CAD build for the part. Positions are in the model's coordinates, mm. Face numbers are marked on the shaded views. A direction names the side the tool comes from. Coordinates: 2 decimals unless noted, no trailing zeros. Write each loop counter-clockwise with the first axis right and the second up, starting at its lowest first coordinate (ties: lowest second). Pieces come first, ordered by that corner, then holes.
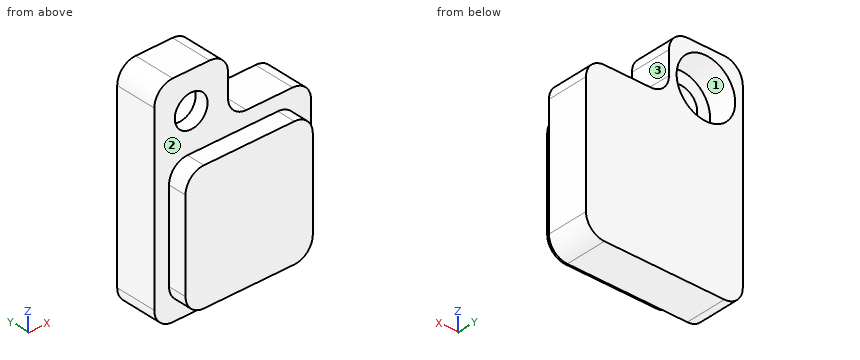
```python
from build123d import *

# Parameters (mm, degrees)
SKETCH1_W                                      = 8.5
SKETCH1_H                                      = 8.5
EXTRUDE1_DEPTH                                 = 2.25
SKETCH7_W                                      = 6.9
SKETCH7_H                                      = 6.9
EXTRUDE5_DEPTH                                 = 1
SKETCH3_W                                      = 4
SKETCH3_H                                      = 2.25
EXTRUDE3_DEPTH                                 = 3.25
CBORE_FOR_0_SOCKET_HEAD_CAP_SCREW1_D           = 1.778
CBORE_FOR_0_SOCKET_HEAD_CAP_SCREW1_CBORE_D     = 3.175
CBORE_FOR_0_SOCKET_HEAD_CAP_SCREW1_CBORE_DEPTH = 1.524
FILLET2_R                                      = 1


with BuildPart() as part:
    # Sketch1 → Extrude1 (new body)
    with BuildSketch(Plane(origin=(0, 0, 0), x_dir=(1, 0, 0), z_dir=(0, 1, 0))):
        Rectangle(SKETCH1_W, SKETCH1_H)
    extrude(amount=EXTRUDE1_DEPTH)

    # Sketch7 → Extrude5 (add)
    with BuildSketch(Plane.XZ):
        Rectangle(SKETCH7_W, SKETCH7_H)
    extrude(amount=EXTRUDE5_DEPTH)

    # Sketch3 → Extrude3 (add)
    with BuildSketch(Plane.XY.offset(4.25)):
        with Locations((-2.25, 1.125)):
            Rectangle(SKETCH3_W, SKETCH3_H)
    extrude(amount=EXTRUDE3_DEPTH)

    # CBORE for #0 Socket Head Cap Screw1 (through all)
    with Locations(Plane(origin=(-2.25, 2.25, 5.5), x_dir=(0, 0, 1), z_dir=(0, 1, 0))):
        with Locations((0, 0)):
            CounterBoreHole(CBORE_FOR_0_SOCKET_HEAD_CAP_SCREW1_D / 2, CBORE_FOR_0_SOCKET_HEAD_CAP_SCREW1_CBORE_D / 2, CBORE_FOR_0_SOCKET_HEAD_CAP_SCREW1_CBORE_DEPTH)

    # Fillet2
    fillet2_edges = [part.edges().sort_by_distance(p)[0] for p in [
        (-3.45, -0.5, -3.45),
        (-4.25, 1.125, -4.25),
        (-3.45, -0.5, 3.45),
        (3.45, -0.5, -3.45),
        (3.45, -0.5, 3.45),
        (4.25, 1.125, -4.25),
        (4.25, 1.125, 4.25),
        (-4.25, 1.125, 7.5),
        (-0.25, 1.125, 7.5),
        (-0.25, 1.125, 4.25),
    ]]
    fillet(fillet2_edges, radius=FILLET2_R)


solid = part.part
```
Item 1: Flat gauge pins, fed straight in: pin 1 Ø1.8 at (x, y) = (2.5, 1.5) entering from +Z; pin 2 Ø1.9 at (x, z) = (-2.25, 5.5) entering from +Y; pin 3 Ø1.6 at (x, z) = (-2.25, 5.5) entering from -Y; pin 4 Ø0.5 at (x, y) = (0, -0.5) entering from -Z. Where does each tip first touch, or does it go through?
Item 2: Saw through at B-B, the plane x = -2.25. Write the cut outline in (y, z).
Item 3: Saw through at C-C, the plane z = 5.5. Write the cut outline in (x, y), and give its area (3 significant figures).
Item 4: Saw through at A-A, the plane y = 0.2. Write the cut outline in (x, z), and give its area (3 significant figures).
Item 5: Which spindle directions (+Z, -Z, +X, -X, +Y, -Y) get a long thin tool onto all of the face, cutting with end or side? Do the marked faces 1, 2 and 3. Say none if no direction does.
Item 6: Wall check: line 1 along X through (y, z) = (1.95, 5.5); line 2 along X through (y, z) = (0.4, 5.5); line 3 along Y through (x, z) = (4, -1.75). Give the ranges that are in metal, low to high.
Item 7: Saw through at D-D, the plane z = -1. Write the cut outline in (x, y).
Working result:
1. pin 1: stops at z = 4.25
1. pin 2: stops at y = 0.73
1. pin 3: passes through
1. pin 4: stops at z = -3.45
2. outline: (-1, -3.45) - (0, -3.45) - (0, -4.25) - (2.25, -4.25) - (2.25, 3.91) - (0.73, 3.91) - (0.73, 4.61) - (0, 4.61) - (0, 3.45) - (-1, 3.45) - close; (0, 6.39) - (0.73, 6.39) - (0.73, 7.09) - (2.25, 7.09) - (2.25, 7.5) - (0, 7.5) - close
3. outline: (-4.25, 0) - (-3.14, 0) - (-3.14, 0.73) - (-3.84, 0.73) - (-3.84, 2.25) - (-4.25, 2.25) - close; (-1.36, 0) - (-0.25, 0) - (-0.25, 2.25) - (-0.66, 2.25) - (-0.66, 0.73) - (-1.36, 0.73) - close
3. area: 2.87 mm2
4. outline: (-4.25, -3.25) arc R1 ccw to (-3.25, -4.25) - (3.25, -4.25) arc R1 ccw to (4.25, -3.25) - (4.25, 3.25) arc R1 ccw to (3.25, 4.25) - (0.75, 4.25) arc R1 cw to (-0.25, 5.25) - (-0.25, 6.5) arc R1 ccw to (-1.25, 7.5) - (-3.25, 7.5) arc R1 ccw to (-4.25, 6.5) - close; hole circle Ø1.78 at (-2.25, 5.5)
4. area: 81.9 mm2
5. face 1: +Y
5. face 2: -Y
5. face 3: +Z, +X, +Y, -Y
6. line 1: x = -4.25 to -3.84, -0.66 to -0.25
6. line 2: x = -4.25 to -3.14, -1.36 to -0.25
6. line 3: y = 0 to 2.25
7. outline: (-4.25, 0) - (-3.45, 0) - (-3.45, -1) - (3.45, -1) - (3.45, 0) - (4.25, 0) - (4.25, 2.25) - (-4.25, 2.25) - close
